For this review, take the finished solid that the model builds, in its own axes (mm). A direction names the side the tool comes from. Coordinates: 2 decimals unless noted, no trailing zeros. Order: outer loops, then holes, each group sorted by start corner. A loop starts at its lowest first (then second) coordinate and runs counter-clockwise, first axis right, second up.
from build123d import *

# Parameters (mm, degrees)
SKETCH1_W           = 7.874
SKETCH1_H           = 38.1
SKETCH2_R           = 65.151
SKETCH2_R_2         = 42.926
BOSS_EXTRUDE2_DEPTH = 7.874
SKETCH4_R           = 5.588
CUT_EXTRUDE1_DEPTH  = 8.874
SKETCH5_R           = 5.588
BOSS_EXTRUDE4_DEPTH = 7.62


with BuildPart() as part:
    # Sketch1 → Revolve1 (revolve)
    with BuildSketch(Plane.XY):
        with Locations((-69.088, 19.05)):
            Rectangle(SKETCH1_W, SKETCH1_H)
    revolve(axis=Axis((0, 92.899450936, 0), (0, -1, 0)))

    # Sketch2 → Boss-Extrude2 (add)
    with BuildSketch(Plane(origin=(0, 0, 0), x_dir=(1, 0, 0), z_dir=(0, 1, 0))):
        Circle(SKETCH2_R)
        Circle(SKETCH2_R_2, mode=Mode.SUBTRACT)
    extrude(amount=BOSS_EXTRUDE2_DEPTH)

    # Sketch4 → Cut-Extrude1 (cut, through all)
    with BuildSketch(Plane(origin=(0, 7.874, 0), x_dir=(1, 0, 0), z_dir=(0, 1, 0))):
        with Locations((0, 54.102)):
            Circle(SKETCH4_R)
        with Locations((38.255891076, 38.255891076)):
            Circle(SKETCH4_R)
        with Locations((54.102, 0)):
            Circle(SKETCH4_R)
        with Locations((38.255891076, -38.255891076)):
            Circle(SKETCH4_R)
        with Locations((0, -54.102)):
            Circle(SKETCH4_R)
        with Locations((-38.255891076, -38.255891076)):
            Circle(SKETCH4_R)
        with Locations((-54.102, 0)):
            Circle(SKETCH4_R)
        with Locations((-38.255891076, 38.255891076)):
            Circle(SKETCH4_R)
    extrude(amount=-CUT_EXTRUDE1_DEPTH, mode=Mode.SUBTRACT)

    # Sketch5 → Boss-Extrude4 (add)
    with BuildSketch(Plane(origin=(0, 38.1, 0), x_dir=(1, 0, 0), z_dir=(0, 1, 0))):
        with BuildLine():
            Line((-54.102, 11.176), (-64.185277323, 11.176))
            ThreePointArc((-64.185277323, 11.176), (-65.151, 0), (-64.185277323, -11.176))
            Line((-64.185277323, -11.176), (-54.102, -11.176))
            ThreePointArc((-54.102, -11.176), (-42.926, 0), (-54.102, 11.176))
        make_face()
        with Locations((-54.102, 0)):
            Circle(SKETCH5_R, mode=Mode.SUBTRACT)
        with BuildLine():
            Line((11.176, 54.102), (11.176, 64.185277323))
            ThreePointArc((11.176, 64.185277323), (0, 65.151), (-11.176, 64.185277323))
            Line((-11.176, 64.185277323), (-11.176, 54.102))
            ThreePointArc((-11.176, 54.102), (0, 42.926), (11.176, 54.102))
        make_face()
        with Locations((0, 54.102)):
            Circle(SKETCH5_R, mode=Mode.SUBTRACT)
        with BuildLine():
            ThreePointArc((65.151, 0), (64.909120329, 5.608823323), (64.185277323, 11.176))
            Line((64.185277323, 11.176), (54.102, 11.176))
            ThreePointArc((54.102, 11.176), (42.926, 0), (54.102, -11.176))
            Line((54.102, -11.176), (64.185277323, -11.176))
            ThreePointArc((64.185277323, -11.176), (64.909120329, -5.608823323), (65.151, 0))
        make_face()
        with Locations((54.102, 0)):
            Circle(SKETCH5_R, mode=Mode.SUBTRACT)
        with BuildLine():
            ThreePointArc((-11.176, -64.185277323), (0, -65.151), (11.176, -64.185277323))
            Line((11.176, -64.185277323), (11.176, -54.102))
            ThreePointArc((11.176, -54.102), (0, -42.926), (-11.176, -54.102))
            Line((-11.176, -54.102), (-11.176, -64.185277323))
        make_face()
        with Locations((0, -54.102)):
            Circle(SKETCH5_R, mode=Mode.SUBTRACT)
    extrude(amount=-BOSS_EXTRUDE4_DEPTH)


solid = part.part
1. Take a section at C-C, the plane y = 33. Give the boundary of the cut face in (x, z) (3 decimals), plus the area to 3 significant figures.
Answer below:
outline: circle Ø146.05 at (0, 0); hole (-64.185, -11.176) arc R65.151 ccw to (-11.176, -64.185) - (-11.176, -54.102) arc R11.176 cw to (11.176, -54.102) - (11.176, -64.185) arc R65.151 ccw to (64.185, -11.176) - (54.102, -11.176) arc R11.176 cw to (54.102, 11.176) - (64.185, 11.176) arc R65.151 ccw to (11.176, 64.185) - (11.176, 54.102) arc R11.176 cw to (-11.176, 54.102) - (-11.176, 64.185) arc R65.151 ccw to (-64.185, 11.176) - (-54.102, 11.176) arc R11.176 cw to (-54.102, -11.176) - close; hole circle Ø11.176 at (-54.102, 0); hole circle Ø11.176 at (0, -54.102); hole circle Ø11.176 at (0, 54.102); hole circle Ø11.176 at (54.102, 0)
area: 4,770 mm2
2. The part is to be moulded in two halves that separate along Z. For faces 1 (the face through (-11.176, 34, 59)), 2 (the face through (0, 30.48, 61)), say which applies: +Z half, -Z half, draft (parallel to the pull), parting line (faces both ways), or undercut.
Answer below:
face 1: undercut
face 2: undercut
3. To check wall thickness, follow L1, parallel to Z at x = 0, y = 35.5 (3 decimals); L2, parallel to Z at x = -44.5, y = 33. State the ranges of each line that lie inside material, in increasing order.
Answer below:
L1: z = -73.025 to -59.69, -48.514 to -42.926, 42.926 to 48.514, 59.69 to 73.025
L2: z = -57.9 to -47.59, -5.72 to 5.72, 47.59 to 57.9
4. Machinability: for faces 3 (the face through (40.944, 3.882, -12.894)), 4 (the face through (61, 30.48, 0)), 5 (the face through (-42.93, 34.34, 0.25)), which of the approach directions +Z, -Z, +X, -X, +Y, -Y give a long, thin tool a straight path to every point of the face, cutting with its end or side? Answer none if there is none.
Answer below:
face 3: +Y, -Y
face 4: none
face 5: +Y
5. Take a section at A-A, the plane z = 0. Give the number of separate pieces and of enclosed holes in the cut face, plus the area to 3 significant figures.
Answer below:
separate pieces: 6
enclosed holes: 0
area: 942 mm2
6. Clearance check with flat-ended pins moving along their axes: pin 1 Ø1.5 at (x, z) = (-42, 17) entering from +Y; pin 2 Ø10 at (x, y) = (14.5, 18.5) entering from -Z; pin 3 Ø10 at (x, z) = (-38.26, 38.26) entering from -Y; pin 4 Ø2 at (y, z) = (9.5, 55.5) entering from +X. State where each tip first meets the part, or that it passes through.
Answer below:
pin 1: stops at y = 7.87
pin 2: stops at z = -72.4
pin 3: passes through
pin 4: stops at x = 48.6
7. Take a section at D-D, the plane x = -15. Give the boundary of the cut face in (y, z).
Answer below:
outline: (0, -71.47) - (38.1, -71.47) - (38.1, -63.4) - (7.87, -63.4) - (7.87, -40.22) - (0, -40.22) - close; (0, 40.22) - (7.87, 40.22) - (7.87, 63.4) - (38.1, 63.4) - (38.1, 71.47) - (0, 71.47) - close
